```python
from build123d import *

# Parameters (mm, degrees)
BOSS_EXTRUDE2_DEPTH = 50
CUT_EXTRUDE2_DEPTH  = 5
FILLET1_R           = 0.5


with BuildPart() as part:
    # Sketch1 → Boss-Extrude2 (new body)
    with BuildSketch(Plane.XY):
        Polygon((0, 0), (0, 25), (20, 25), (50, 15), (50, 0), align=None)
    extrude(amount=BOSS_EXTRUDE2_DEPTH)

    # Sketch3 → Cut-Extrude2 (cut)
    with BuildSketch(Plane(origin=(9.5, 28.5, 0), x_dir=(0.948683298, -0.316227766, 0), z_dir=(0.316227766, 0.948683298, 0))):
        with BuildLine():
            Line((17.690748412, -15), (17.690748412, -30))
            ThreePointArc((17.690748412, -30), (22.690748412, -35), (27.690748412, -30))
            Line((27.690748412, -30), (27.690748412, -15))
            ThreePointArc((27.690748412, -15), (22.690748412, -10), (17.690748412, -15))
        make_face()
    extrude(amount=-CUT_EXTRUDE2_DEPTH, mode=Mode.SUBTRACT)

    # Fillet1
    fillet1_edges = [part.edges().sort_by_distance(p)[0] for p in [
        (31.026334039, 21.32455532, 10),
        (26.282917549, 22.90569415, 22.5),
        (31.026334039, 21.32455532, 35),
        (35.769750529, 19.74341649, 22.5),
    ]]
    fillet(fillet1_edges, radius=FILLET1_R)


solid = part.part
```
Input: part model. Units: mm. Frame: model coordinates. A direction names the side the tool comes from. Round coordinates to 2 decimals unless told otherwise and drop trailing zeros. Loops run counter-clockwise (first coordinate to the right, second up) from the corner with the lowest first, then second, coordinate; pieces in that order, holes last. Notation, with made-up numbers: (-39, -3) - (-30, -3) arc R10 cw to (-30, 8) - close; hole circle Ø5 at (89, 45.25). An arc over 180 degrees is marked (long way). One line per item, written item: value. Start each with the question number.
(1) Contact query for a flat-ended pin moving along its axis: P1, Ø12, axis at y = 7, z = 17.5, coming from the -X side. Output: stop coordinate, or through.
(2) Ray query, line 1 (Z direction, x = 29, y = 18.5); line 2 (Y direction, x = 42.5, z = 17.5); line 3 (Y direction, x = 40.5, z = 42.5). Return the intervals inside material, ascending. Write a range as [from, to].
(3) Draft query along Z for faces 4 (the flat face through (50, 8, 25)), 5 (the flat face through (25, 13, 0)), 6 (the cylindrical face through (30.1, 18.8, 35)), 7 (the flat face through (25, 13, 50)). Return one class per face: +Z half, -Z half, draft (parallel to the pull), parting line (faces both ways), or undercut.
(4) Section C-C, the plane z = 28.5. Return loops of the section in (x, y), plus the area to 3 significant figures.
(5) Section D-D, the plane x = 45.5. Return loops of the section in (y, z).
(6) Access query for faces 1 (the flat face through (25.423, 20.327, 22.395)), 2 (the flat face through (25, 0, 25)), 3 (the flat face through (34.91, 17.16, 22.6)). Directions: +Z, -Z, +X, -X, +Y, -Y. A direction counts if a zero-diameter tool reaches every point of the face in a straight line with its end or side. Return the directions, or none.
(7) Section A-A, the plane z = 41.5. Return loops of the section in (x, y), plus the area to 3 significant figures.
(8) Section B-B, the plane x = 38. Return loops of the section in (y, z).
Results below:
1. P1: x = 0
2. line 1: [0, 10.11], [34.89, 50]
2. line 2: [0, 17.5]
2. line 3: [0, 18.17]
3. face 4: draft
3. face 5: -Z half
3. face 6: undercut
3. face 7: +Z half
4. outline: (0, 0) - (50, 0) - (50, 15) - (36.24, 19.59) arc R0.5 ccw to (35.61, 19.27) - (34.19, 15) - (24.7, 18.16) - (26.12, 22.43) arc R0.5 ccw to (25.81, 23.06) - (20, 25) - (0, 25) - close
4. area: 1,050 mm^2
5. outline: (0, 0) - (16.5, 0) - (16.5, 50) - (0, 50) - close
6. face 1: none
6. face 2: +Z, -Z, +X, -X, -Y
6. face 3: +Y
7. outline: (0, 0) - (50, 0) - (50, 15) - (20, 25) - (0, 25) - close
7. area: 1,100 mm^2
8. outline: (0, 0) - (19, 0) - (19, 50) - (0, 50) - close
